Geometry: final body of the model. Coordinates: model frame, mm. Face numbers are marked on the shaded views. A direction names the side the tool comes from. Round coordinates to 2 decimals unless told otherwise and drop trailing zeros. Loops run counter-clockwise (first coordinate to the right, second up) from the corner with the lowest first, then second, coordinate; pieces in that order, holes last. Notation, with made-up numbers: (-27.75, 36.5) - (-4.75, 36.5) arc R28 cw to (-4.75, 64.5) - close; hole circle Ø11 at (-3.75, 8.25). An arc over 180 degrees is marked (long way). Return JSON: item names as keys, results as strings. Group by question number.
1. Section C-C on x = -82.55. Return loops of the section in (y, z) (1 decimal), and give its area (3 significant figures).
2. Section B-B on y = 25.4. Return loops of the section in (x, z).
3. Section A-A on z = 0. Count the separate pieces of the cut face and the enclosed holes in it, and give its area (3 significant figures).
4. Section D-D on x = -20. Return loops of the section in (y, z) (3 decimals).
5. First-contact query: pin 1 Ø15 at (x, z) = (-92, -0.5) entering from -Y (3 decimals); pin 2 Ø1 at (y, z) = (183, -16.5) entering from -X; pin 3 Ø5.5 at (x, z) = (-82.55, 0) entering from -Y; pin 4 Ø15.5 at (y, z) = (25.4, 0) entering from +X. Flat tips, straight axial feed; report the tip coordinate or a pass-through.
6. Set-up query: the marked faces 1, 2 and 3. Return all of +Z, -Z, +X, -X, +Y, -Y with unobstructed straight access to the full face (end or side cutting, diameter ignored); none if empty.
7. Material intervals for probe 1 along Z at (x, y) = (-2, 25); probe 2 along X at (y, z) = (196.5, -10); probe 3 along Y at (x, z) = (-90, -15) (3 decimals), sorted ascending.
from build123d import *

# Parameters (mm, degrees)
F1_DEPTH = 25.4
F2_R     = 4.7625
F3_DEPTH = 50.801
F4_R     = 4.826
F5_DEPTH = 209.551


with BuildPart() as f1:
    # F0 (on Top) → F1 (new body, symmetric)
    with BuildSketch(Plane.XY):
        Polygon((-6.35, 219.075), (-6.35, 0), (0, 0), (0, 225.425), (-203.2, 225.425), (-203.2, 269.875), (-209.55, 269.875), (-209.55, 219.075), align=None)
    extrude(amount=F1_DEPTH, both=True)

    # F2 (on face) → F3 (cut, through all)
    with BuildSketch(Plane.XZ.offset(-219.075)):
        with Locations((-82.55, 0)):
            Circle(F2_R)
    extrude(amount=-F3_DEPTH, mode=Mode.SUBTRACT)

    # F4 (on face) → F5 (cut, through all)
    with BuildSketch(Plane.YZ):
        with Locations((25.4, 0)):
            Circle(F4_R)
    extrude(amount=-F5_DEPTH, mode=Mode.SUBTRACT)


solid = f1.part
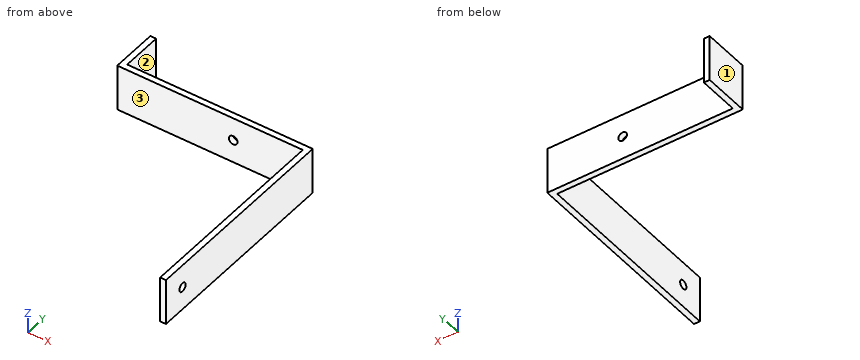
Taken from the geometry:
{
 "1": {"outline": "(219.1, -25.4) - (225.4, -25.4) - (225.4, -4.8) - (219.1, -4.8) - close; (219.1, 4.8) - (225.4, 4.8) - (225.4, 25.4) - (219.1, 25.4) - close", "area": "262 mm2"},
 "2": {"outline": "(-6.35, -25.4) - (0, -25.4) - (0, -4.83) - (-6.35, -4.83) - close; (-6.35, 4.83) - (0, 4.83) - (0, 25.4) - (-6.35, 25.4) - close"},
 "3": {"separate pieces": "3", "enclosed holes": "0", "area": "2,880 mm2"},
 "4": {"outline": "(219.075, -25.4) - (225.425, -25.4) - (225.425, 25.4) - (219.075, 25.4) - close"},
 "5": {"pin 1": "y = 219.075", "pin 2": "x = -6.35", "pin 3": "through", "pin 4": "x = 0"},
 "6": {"face 1": "+Z, -Z, -X, +Y, -Y", "face 2": "+Z, -Z, +X, +Y", "face 3": "+Z, -Z, -X, -Y"},
 "7": {"probe 1": "-25.4 to -4.81, 4.81 to 25.4", "probe 2": "-6.35 to 0", "probe 3": "219.075 to 225.425"}
}
